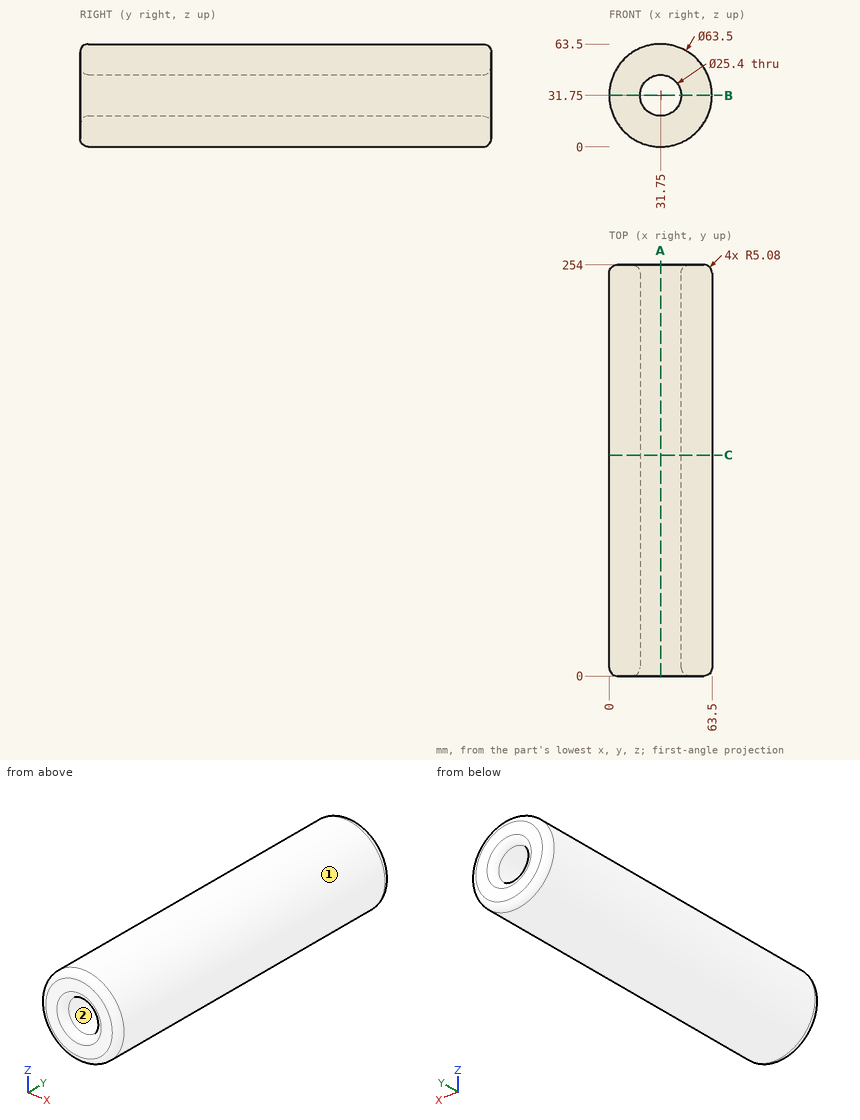
Geometry: see drawing. Coordinates: mm, zero at the bounding-box minimum. Coordinates: 2 decimals unless noted, no trailing zeros. Write each loop counter-clockwise with the first axis right and the second up, starting at its lowest first coordinate (ties: lowest second). Pieces come first, ordered by that corner, then holes. Notation, with made-up numbers: M 50.5,20 L 77.5,20 A25 ccw 77.5,37 Z; hole C 37.25,69 d5. An arc over 180 degrees is marked long. Use CSV: the item, a comma, the result in double quotes. Start each with the question number.
1. Mould query, pull axis X, two halves, no side actions, for the marked faces 1 and 2. Classes: pulls with the +X half, pulls with the -X half, needs draft (parallel to the pull), parting line crosses it, or undercut.
2. Cut plane A-A on x = 31.75. Return the cut outline in (y, z), plus the area to 3 significant figures.
3. Cut plane B-B on z = 31.75. Return the cut outline in (x, y), plus the area to 3 significant figures.
4. Cut plane C-C on y = 136.5. Return the cut outline in (x, z), plus the area to 3 significant figures.
5. Ray query, probe 1 along Z at (x, y) = (31.75, 189); probe 2 along X at (y, z) = (106.5, 49); probe 3 along X at (y, z) = (48, 37). Return the intervals inside material, ascending.
6. First-contact query: P1, Ø12, axis at x = 52, y = 127.5, coming from the -Z side; P2, Ø1.5, axis at y = 127, z = 53, coming from the +X side; P3, Ø3, axis at y = 35, z = 29, coming from the -X side. Flat tips, straight axial feed; report the tip coordinate or a pass-through.
Entries:
1,face 1,"parting line crosses it"
1,face 2,"undercut"
2,outline,"M 0,5.08 A5.08 ccw 5.08,0 L 248.92,0 A5.08 ccw 254,5.08 L 254,13.97 A5.08 ccw 248.92,19.05 L 5.08,19.05 A5.08 ccw 0,13.97 Z; M 0,49.53 A5.08 ccw 5.08,44.45 L 248.92,44.45 A5.08 ccw 254,49.53 L 254,58.42 A5.08 ccw 248.92,63.5 L 5.08,63.5 A5.08 ccw 0,58.42 Z"
2,area,"9,630 mm²"
3,outline,"M 0,5.08 A5.08 ccw 5.08,0 L 13.97,0 A5.08 ccw 19.05,5.08 L 19.05,248.92 A5.08 ccw 13.97,254 L 5.08,254 A5.08 ccw 0,248.92 Z; M 44.45,5.08 A5.08 ccw 49.53,0 L 58.42,0 A5.08 ccw 63.5,5.08 L 63.5,248.92 A5.08 ccw 58.42,254 L 49.53,254 A5.08 ccw 44.45,248.92 Z"
3,area,"9,630 mm²"
4,outline,"C 31.75,31.75 d63.5; hole C 31.75,31.75 d25.4"
4,area,"2,660 mm²"
5,probe 1,"0 to 19.05, 44.45 to 63.5"
5,probe 2,"5.09 to 58.41"
5,probe 3,"0.44 to 20.19, 43.31 to 63.06"
6,P1,"z = 3.38"
6,P2,"x = 55.99"
6,P3,"x = 0.02"
